For this review, use the dimensioned drawing (mm, ordinates from the lowest corner) and the shaded views. Give positions to 0.01 mm unless a question says otherwise; leave off trailing zeros. Loops run counter-clockwise (first coordinate to the right, second up) from the corner with the lowest first, then second, coordinate; pieces in that order, holes last. Notation, with made-up numbers: (49, -11.75) - (56, -11.75) arc R27 ccw to (56, 11.25) - close; hole circle Ø4 at (71, 69). An arc over 180 degrees is marked (long way). Put each result on its own line as item: value.
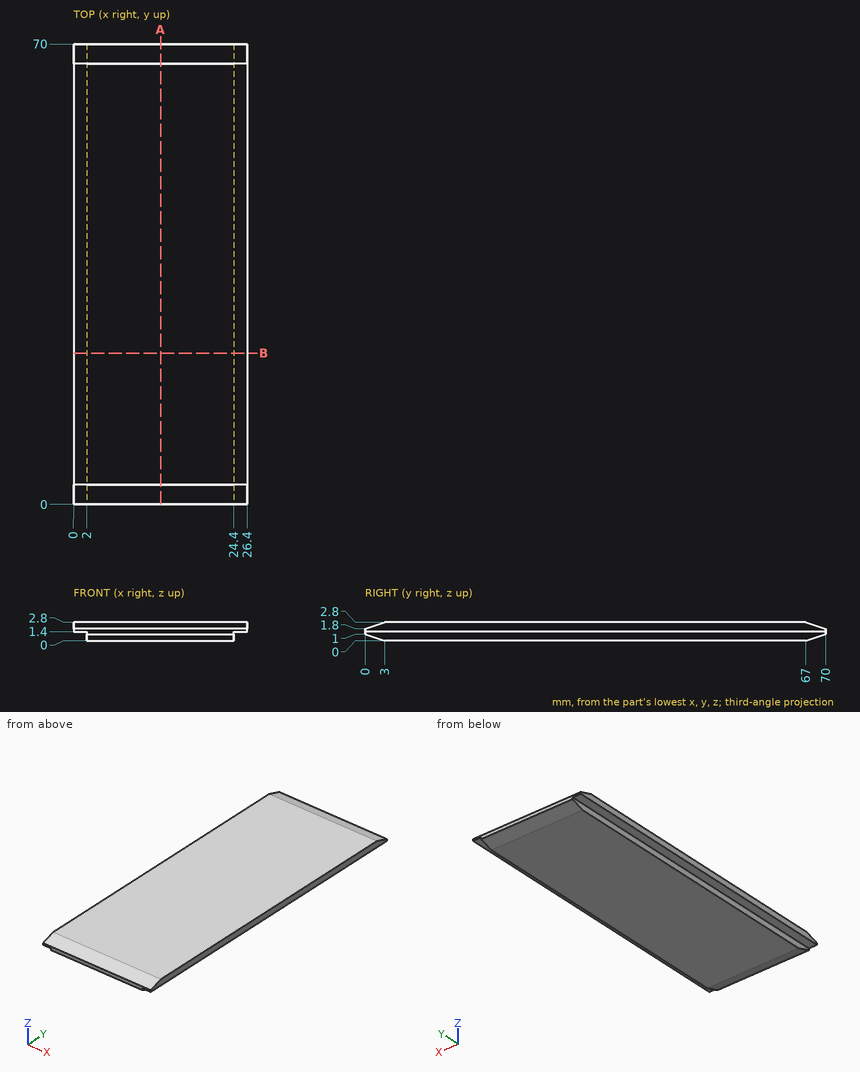
1) Wall thickness on line 1 (X direction, y = 46, z = 0.5); line 2 (Z direction, x = 1.75, y = 18): over which ranges is each line inside the solid? List them lowest first.
Geometry check:
line 1: x = 2 to 24.4
line 2: z = 1.4 to 2.8
2) Insertion check: pin 1 Ø1.1 at (y, z) = (33.5, 0.5) entering from -X; pin 2 Ø1 at (y, z) = (7, 1) entering from -X; pin 3 Ø1.6 at (x, y) = (0.5, 29) entering from -Z. Each pin has a flat end and moves straight along its axis. Give the tip position at first contact, or say it passes through.
Geometry check:
pin 1: stops at x = 2
pin 2: stops at x = 0
pin 3: stops at z = 1.4
3) Take a section at A-A on x = 13.25. State the section outline as (y, z) points.
Geometry check:
outline: (0, 1) - (3, 0) - (67, 0) - (70, 1) - (70, 1.8) - (67, 2.8) - (3, 2.8) - (0, 1.8) - close
4) Take a section at B-B on y = 23. State the section outline as (x, z) points.
Geometry check:
outline: (0, 1.4) - (2, 1.4) - (2, 0) - (24.4, 0) - (24.4, 1.4) - (26.4, 1.4) - (26.4, 2.8) - (0, 2.8) - close
